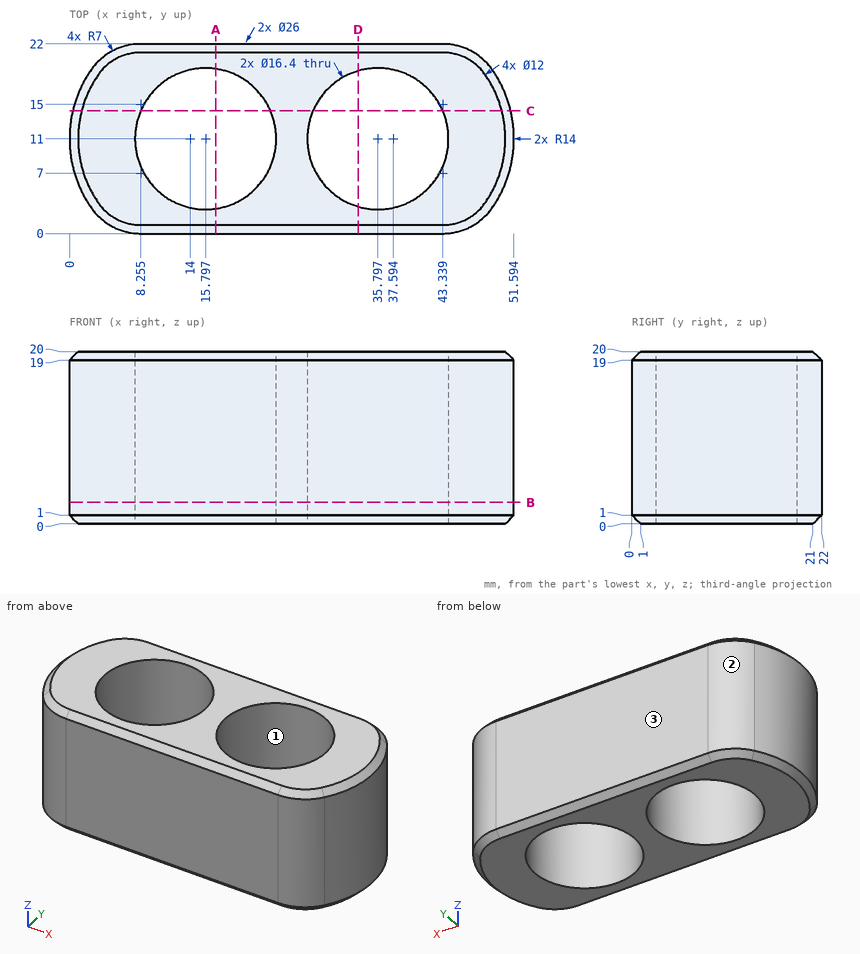
Print and shaded views of the part. All mm, measured from the part's lowest x, y and z. Give positions to 0.01 mm unless a question says otherwise; leave off trailing zeros. Loops run counter-clockwise (first coordinate to the right, second up) from the corner with the lowest first, then second, coordinate; pieces in that order, holes last.
1) Wall check: line 1 (X direction, y = 8, z = 2) (1 decimal); line 2 (X direction, y = 10, z = 17.25) (1 decimal); line 3 (Y direction, x = 39.5, z = 18) (1 decimal). Give the ranges that are in metal, low to high.
2) Flat gauge pins, fed straight in: pin 1 Ø5 at (x, y) = (43.5, 4) entering from -Z; pin 2 Ø1 at (y, z) = (2.5, 12) entering from +X; pin 3 Ø2 at (y, z) = (4, 15.5) entering from -X. Where does each tip first touch, or does it go through?
3) Saw through at D-D (x = 33.5). Write the cut outline in (y, z), plus the area to 3 significant figures.
4) Saw through at B-B (z = 2.5). Write the cut outline in (x, y) (1 decimal), plus the area to 3 significant figures.
5) Pull direction X, two halves, no side cores. Call the marked faces 1, 2 and 3: +X half, -X half, draft (parallel to the pull), parting line (faces both ways), or undercut.
6) Saw through at C-C (y = 14.25). Count the separate pieces of the cut face and the enclosed holes in it, plus the area to 3 significant figures.
7) Saw through at A-A (x = 17). Write the cut outline in (y, z).
Answer block:
1. line 1: x = 0.3 to 8.2, 23.4 to 28.2, 43.4 to 51.3
1. line 2: x = 0 to 7.7, 23.9 to 27.7, 43.9 to 51.6
1. line 3: y = 0 to 3.7, 18.3 to 22
2. pin 1: stops at z = 0
2. pin 2: stops at x = 49.08
2. pin 3: stops at x = 1.35
3. outline: (0, 1) - (1, 0) - (3.13, 0) - (3.13, 20) - (1, 20) - (0, 19) - close; (18.87, 0) - (21, 0) - (22, 1) - (22, 19) - (21, 20) - (18.87, 20) - close
3. area: 123 mm2
4. outline: (2.5, 3) arc R7 ccw to (8.3, 0) - (43.3, 0) arc R7 ccw to (49.1, 3) arc R14 ccw to (49.1, 19) arc R7 ccw to (43.3, 22) - (8.3, 22) arc R7 ccw to (2.5, 19) arc R14 ccw to start; hole circle Ø16.4 at (15.8, 11); hole circle Ø16.4 at (35.8, 11)
4. area: 636 mm2
5. face 1: undercut
5. face 2: -X half
5. face 3: draft
6. separate pieces: 3
6. enclosed holes: 0
6. area: 412 mm2
7. outline: (0, 1) - (1, 0) - (2.89, 0) - (2.89, 20) - (1, 20) - (0, 19) - close; (19.11, 0) - (21, 0) - (22, 1) - (22, 19) - (21, 20) - (19.11, 20) - close
